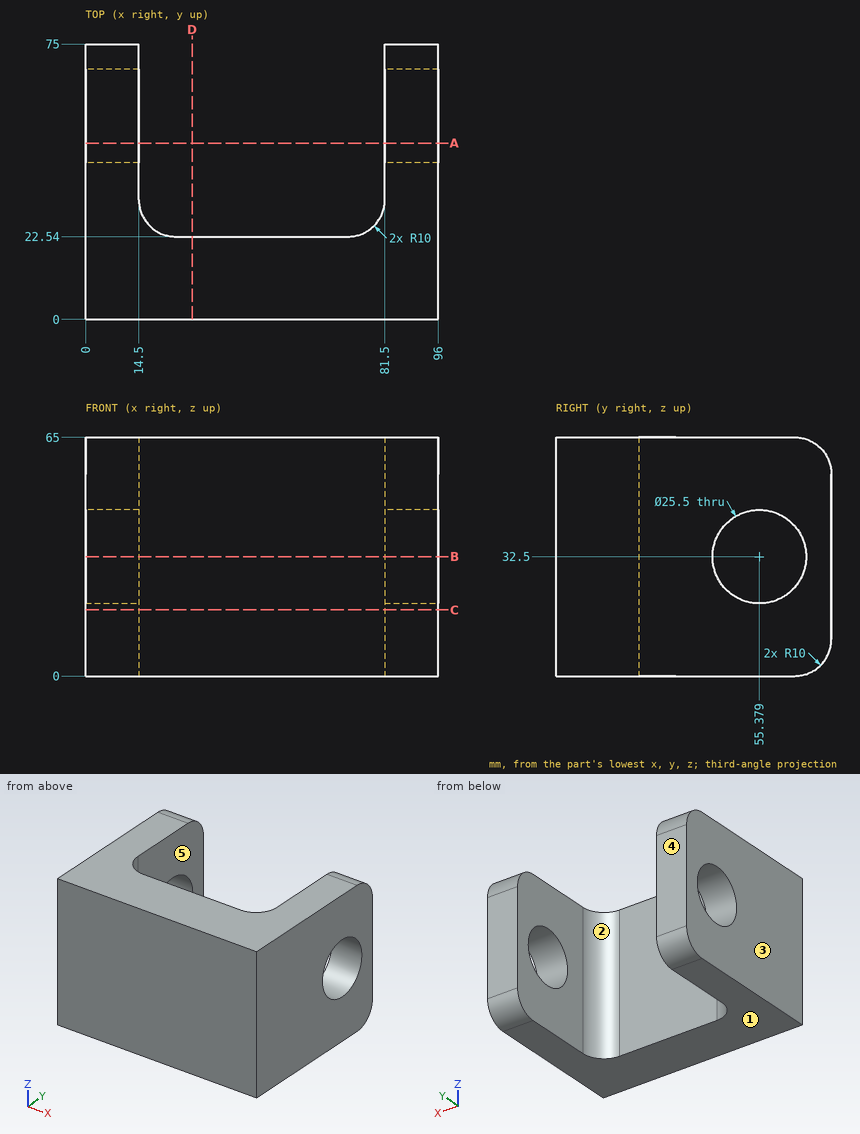
Design review of the part shown in the three views and the two pictorial views. Dimensions are in mm from the part's minimum x, y and z. A direction names the side the tool comes from. Round coordinates to 2 decimals unless told otherwise and drop trailing zeros. Order: outer loops, then holes, each group sorted by start corner. A loop starts at its lowest first (then second) coordinate and runs counter-clockwise, first axis right, second up. Notation, with made-up numbers: (17.5, -28.5) - (64.5, -28.5) arc R8 cw to (64.5, -21.5) - close; hole circle Ø1 at (22, 9). An arc over 180 degrees is marked (long way). Answer in a Markdown table with one row per item.
(1) Take a section at A-A on y = 48. Write out the cut boundary in (x, z).
Result set:
| item | result |
|---|---|
| outline | (0, 0) - (14.5, 0) - (14.5, 22.1) - (0, 22.1) - close; (0, 42.9) - (14.5, 42.9) - (14.5, 65) - (0, 65) - close; (81.5, 0) - (96, 0) - (96, 22.1) - (81.5, 22.1) - close; (81.5, 42.9) - (96, 42.9) - (96, 65) - (81.5, 65) - close |
(2) Clearance check with flat-ended pins moving along their axes: P1, Ø8, axis at x = 38.5, z = 48.5, coming from the +Y side; P2, Ø20.5, axis at y = 55.38, z = 32.5, coming from the +X side. State where each tip first meets the part, or that it passes through.
Result set:
| item | result |
|---|---|
| P1 | stops at y = 22.54 |
| P2 | passes through |
(3) Machinability: for the marked faces 1 and 2, which of the approach directions +Z, -Z, +X, -X, +Y, -Y give a long, thin tool a straight path to every point of the face, cutting with its end or side? Answer none if there is none.
Result set:
| item | result |
|---|---|
| face 1 | -Z, +X, -X, +Y, -Y |
| face 2 | +Z, -Z, +Y |
(4) Take a section at D-D on x = 29. Write out the cut boundary in (y, z).
Result set:
| item | result |
|---|---|
| outline | (0, 0) - (22.54, 0) - (22.54, 65) - (0, 65) - close |
(5) Mouldability with a two-part tool opening along X and no side actions: class the marked faces 3, 4 and 5 as released by +X, released by -X, zero draft, split by the parting line, or undercut.
Result set:
| item | result |
|---|---|
| face 3 | released by -X |
| face 4 | zero draft |
| face 5 | undercut |
(6) For line 1 (X direction, y = 69, z = 7); line 2 (Y direction, x = 84.5, z = 32.5); line 3 (Y direction, x = 68.5, z = 39), list the stretches that pass through material, from the lowest coordinate up. Write a range as from..to.
Result set:
| item | result |
|---|---|
| line 1 | x = 0..14.5, 81.5..96 |
| line 2 | y = 0..42.63, 68.13..75 |
| line 3 | y = 0..22.54 |
(7) Take a section at B-B on z = 32.5. Write out the cut boundary in (x, y).
Result set:
| item | result |
|---|---|
| outline | (0, 0) - (96, 0) - (96, 42.63) - (81.5, 42.63) - (81.5, 32.54) arc R10 cw to (71.5, 22.54) - (24.5, 22.54) arc R10 cw to (14.5, 32.54) - (14.5, 42.63) - (0, 42.63) - close; (0, 68.13) - (14.5, 68.13) - (14.5, 75) - (0, 75) - close; (81.5, 68.13) - (96, 68.13) - (96, 75) - (81.5, 75) - close |
(8) Take a section at C-C on z = 18. Write out the cut boundary in (x, y).
Result set:
| item | result |
|---|---|
| outline | (0, 0) - (96, 0) - (96, 75) - (81.5, 75) - (81.5, 32.54) arc R10 cw to (71.5, 22.54) - (24.5, 22.54) arc R10 cw to (14.5, 32.54) - (14.5, 75) - (0, 75) - close |
